Check sheet for the modelled part. Datum: model origin and axes. Units: mm. A direction names the side the tool comes from. Coordinates: 2 decimals unless noted, no trailing zeros. Loops run counter-clockwise (first coordinate to the right, second up) from the corner with the lowest first, then second, coordinate; pieces in that order, holes last. Notation, with made-up numbers: M 3,-8 L 47,-8 A27 cw 47,20 Z; hole C 33,-7.5 d10. An arc over 180 degrees is marked long. Return JSON: item names as keys, results as strings.
Autodesk Inventor part; units mm, degrees
ref_plane "YZ Plane" through (0, 0, 0) normal (1, 0, 0) x (0, 1, 0)
ref_plane "XZ Plane" through (0, 0, 0) normal (0, 1, 0) x (-1, 0, 0)
ref_plane "XY Plane" through (0, 0, 0) normal (0, 0, 1) x (1, 0, 0)
sketch "Sketch1" plane through (0, 0, 0) normal (0, 0, 1) x (1, 0, 0)
  line L0 (0, 0) -> (25.4, 0)
  line L1 (25.4, 0) -> (25.4, 25.4)
  line L2 (25.4, 25.4) -> (0, 25.4)
  line L3 (0, 25.4) -> (0, 0)
  dimension "d0" = 25.4
  dimension "d1" = 25.4
extrude "Extrusion1" add sketch "Sketch1" along normal blind 279.4
shell "Shell1" thickness 1.5875 removed faces 2 at (8.4667, 16.9333, 0) at (8.4667, 16.9333, 279.4)
sketch "Sketch2" plane through (25.4, 0, 0) normal (1, 0, 0) x (0, 0, -1)
  line L0 (-279.4, 25.4) -> (-279.4, 0)
  line L1 (0, 0) -> (0, 25.4)
  line L2 (0, 25.4) -> (-279.4, 25.4)
  line L3 (-279.4, 0) -> (-279.4, 25.4)
  line L4 (-254, 25.4) -> (-279.4, 25.4)
  line L5 (-279.4, 0) -> (-254, 25.4)
  line L6 (0, 25.4) -> (0, 0)
  line L7 (-25.4, 25.4) -> (0, 0)
  line L8 (-25.4, 25.4) -> (0, 25.4)
  dimension "d5" = 25.4
  dimension "d6" = 25.4
extrude "Extrusion2" cut sketch "Sketch2" against normal through all
sketch "Sketch3" plane through (0, 0, 279.4) normal (0, -1, 0) x (1, 0, 0)
  line L0 (25.4, 0) -> (0, 0)
  line L1 (0, -279.4) -> (25.4, -279.4)
  line L2 (25.4, -279.4) -> (25.4, 0)
  circle A0 centre (12.7, -12.7) radius 3.175
  circle A1 centre (12.7, -266.7) radius 3.175
  dimension "d9" = 6.35
  dimension "d10" = 12.7
  dimension "d11" = 12.7
  dimension "d12" = 12.7
  dimension "d13" = 12.7
extrude "Extrusion3" cut sketch "Sketch3" against normal through all
sketch "Sketch4" plane through (25.4, 0, 279.4) normal (1, 0, 0) x (0, 0, -1)
  circle A0 centre (20.2966, 9.5234) radius 0.9528
extrude "Extrusion4" cut sketch "Sketch4" against normal up to next
properties part number "Frame_LowerCrossSupport" material "Aluminum-6061"
1) Section check B-B on z = 266.7. Record the cut outline in (x, y) (1 decimal).
Answers:
{"outline": "M 0,0 L 9.5,0 L 9.5,1.6 L 1.6,1.6 L 1.6,12.7 L 0,12.7 Z; M 15.9,0 L 25.4,0 L 25.4,12.7 L 23.8,12.7 L 23.8,1.6 L 15.9,1.6 Z"}
2) Go/stop test with flat-tipped pins: pin 1 Ø4 at (x, y) = (22, 5) entering from +Z; pin 2 Ø5.5 at (x, z) = (12.7, 12.7) entering from -Y. Record where each tip stops, or that it passes through.
Answers:
{"pin 1": "z = 275.25", "pin 2": "through"}
3) Section check A-A on x = 12.7. Record the cut outline in (y, z) (1 decimal), then the cut area to 3 significant figures.
Answers:
{"outline": "M 0,0 L 1.6,1.6 L 1.6,9.5 L 0,9.5 Z; M 0,15.9 L 1.6,15.9 L 1.6,263.5 L 0,263.5 Z; M 0,269.9 L 1.6,269.9 L 1.6,277.8 L 0,279.4 Z; M 23.8,23.8 L 25.4,25.4 L 25.4,254 L 23.8,255.6 Z", "area": "786 mm²"}
4) Set-up check for faces 5 (the face through (24, 13, 13)), 6 (the face through (1.588, 13, 138)): record each of +Z, -Z, +X, -X, +Y, -Y from which the full face is reachable in a straight line by a thin tool's end or side.
Answers:
{"face 5": "-Z, +X, -X, +Y", "face 6": "+Z, -Z"}
5) Section check D-D on z = 18.5. Record the cut outline in (x, y).
Answers:
{"outline": "M 0,0 L 25.4,0 L 25.4,18.5 L 23.81,18.5 L 23.81,1.59 L 1.59,1.59 L 1.59,18.5 L 0,18.5 Z"}
6) Scan lines: line 1 along Y through (x, z) = (4, 173.5); line 2 along Z through (x, y) = (12.7, 0.75) (3 decimals). Record each from-to range of solid material in increasing order. Write a range as [from, to].
Answers:
{"line 1": "[0, 1.59], [23.81, 25.4]", "line 2": "[0.75, 9.525], [15.875, 263.525], [269.875, 278.65]"}
7) Section check C-C on z = 148.5. Record the cut outline in (x, y).
Answers:
{"outline": "M 0,0 L 25.4,0 L 25.4,25.4 L 0,25.4 Z; hole M 1.59,1.59 L 23.81,1.59 L 23.81,23.81 L 1.59,23.81 Z"}
8) Draft check along Z on faces 1 (the face through (12.29, 0.78, 269.85)), 2 (the face through (24, 12.6, 266.8)), 3 (the face through (13, 23.812, 138)), 4 (the face through (10.18, 0.78, 10.77)). Enter one of: +Z half, -Z half, draft (parallel to the pull), parting line (faces both ways), or undercut.
Answers:
{"face 1": "undercut", "face 2": "+Z half", "face 3": "draft", "face 4": "undercut"}
